Can you work these out from the model? Positions are in its coordinate system, mm. Face numbers are marked on the shaded views. A direction names the side the tool comes from. Give positions to 0.01 mm unless a question says otherwise; leave off trailing zeros. Order: outer loops, then holes, each group sorted by start corner. A loop starts at its lowest first (then second) coordinate and runs counter-clockwise, first axis right, second up. Notation, with made-up numbers: M 75,-29 L 108,-29 A5 cw 108,-22 Z; hole C 1.5,2.5 d1. An arc over 180 degrees is marked long. Use one line per item in the form item = value. Start each with the question number.
1. I want a section at A-A, the plane z = 0. List the corners of the cut face in (x, y) for me.
2. We'd pull the mould along Z, two halves only. Please class the marked faces 1, 2 and 3: +Z half, -Z half, draft (parallel to the pull), parting line (faces both ways), or undercut.
3. I need wall thicknesses on L1, parallel to X at y = 0.65, z = 0; L2, parallel to X at y = 2.9, z = 0; L3, parallel to X at y = 11.5, z = 0. Which ranges of each line are inside material? Lowest first, please.
4. I want a section at D-D, the plane z = 6.5. List the corners of the cut face in (x, y) for me, and give its area (3 significant figures).
5. I want a section at B-B, the plane x = 0. List the corners of the cut face in (y, z) for me, and give its area (3 significant figures).
6. I want a section at C-C, the plane x = 5.5. List the corners of the cut face in (y, z) for me, and give its area (3 significant figures).
7. Will these pins go through, and if not, where does the flat tip stop? P1, Ø5, axis at x = 0, z = 6, coming from the +Y side; P2, Ø1.5, axis at x = -2.5, y = 17, coming from the +Z side; P3, Ø6, axis at y = 11, z = -5, coming from the -X side.
8. For the marked faces 4, 5 and 6, which set-ups out of +Z, -Z, +X, -X, +Y, -Y let a thin tool reach every point of the face, with its end or its side?
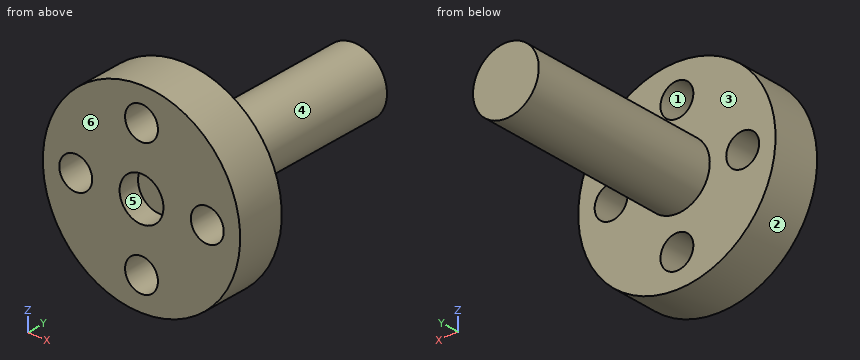
```python
from build123d import *

# Parameters (mm, degrees)
SKETCH_1_R          = 9
EXTRUDE_1_DEPTH     = 4.5
SKETCH_2_R          = 2
CUT_EXTRUDE_1_DEPTH = 2
SKETCH_3_R          = 1.5
CUT_EXTRUDE_2_DEPTH = 14.5
SKETCH_4_R          = 3
EXTRUDE_2_DEPTH     = 18.5


with BuildPart() as part:
    # 草图1 → 凸台-拉伸1 (new body)
    with BuildSketch(Plane(origin=(0, 0, 0), x_dir=(1, 0, 0), z_dir=(0, 1, 0))):
        with Locations(Location((0, 0, 0), (0, 0, 270))):
            Circle(SKETCH_1_R)
    extrude(amount=EXTRUDE_1_DEPTH)

    # 草图2 → 切除-拉伸1 (cut)
    with BuildSketch(Plane.XZ):
        with Locations(Location((0, 0, 0), (0, 0, 270))):
            Circle(SKETCH_2_R)
    extrude(amount=-CUT_EXTRUDE_1_DEPTH, mode=Mode.SUBTRACT)

    # 草图3 → 切除-拉伸2 (cut, through all)
    with BuildSketch(Plane.XZ):
        with Locations(Location((0, 6, 0), (0, 0, 270))):
            Circle(SKETCH_3_R)
        with Locations(Location((6, 0, 0), (0, 0, 270))):
            Circle(SKETCH_3_R)
        with Locations(Location((0, -6, 0), (0, 0, 270))):
            Circle(SKETCH_3_R)
        with Locations(Location((-6, 0, 0), (0, 0, 270))):
            Circle(SKETCH_3_R)
    extrude(amount=-CUT_EXTRUDE_2_DEPTH, mode=Mode.SUBTRACT)

    # 草图4 → 凸台-拉伸2 (add)
    with BuildSketch(Plane(origin=(0, 4.5, 0), x_dir=(1, 0, 0), z_dir=(0, 1, 0))):
        with Locations(Location((0, 0, 0), (0, 0, 270))):
            Circle(SKETCH_4_R)
    extrude(amount=EXTRUDE_2_DEPTH)


solid = part.part
```
Check result:
q1.outline = M -9,0 L -7.5,0 L -7.5,4.5 L -9,4.5 Z; M -4.5,0 L -2,0 L -2,2 L 2,2 L 2,0 L 4.5,0 L 4.5,4.5 L 3,4.5 L 3,23 L -3,23 L -3,4.5 L -4.5,4.5 Z; M 7.5,0 L 9,0 L 9,4.5 L 7.5,4.5 Z
q2.face_1 = undercut
q2.face_2 = parting line
q2.face_3 = draft
q3.L1 = -9 to -7.5, -4.5 to -2, 2 to 4.5, 7.5 to 9
q3.L2 = -9 to -7.5, -4.5 to 4.5, 7.5 to 9
q3.L3 = -3 to 3
q4.outline = M -6.22,0 L -1.41,0 L -1.41,4.5 L -6.22,4.5 Z; M 1.41,0 L 6.22,0 L 6.22,4.5 L 1.41,4.5 Z
q4.area = 43.3 mm2
q5.outline = M 0,-9 L 4.5,-9 L 4.5,-7.5 L 0,-7.5 Z; M 0,-4.5 L 4.5,-4.5 L 4.5,-3 L 23,-3 L 23,3 L 4.5,3 L 4.5,4.5 L 0,4.5 L 0,2 L 2,2 L 2,-2 L 0,-2 Z; M 0,7.5 L 4.5,7.5 L 4.5,9 L 0,9 Z
q5.area = 157 mm2
q6.outline = M 0,-7.12 L 4.5,-7.12 L 4.5,-1.41 L 0,-1.41 Z; M 0,1.41 L 4.5,1.41 L 4.5,7.12 L 0,7.12 Z
q6.area = 51.4 mm2
q7.P1 = 4.5
q7.P2 = 2.44
q7.P3 = -2.24
q8.face_4 = +Y
q8.face_5 = -Y
q8.face_6 = +Z, -Z, +X, -X, -Y
